Build history of the part. All positions in model axes, mm. A direction names the side the tool comes from. Coordinates: 2 decimals unless noted, no trailing zeros. Order: outer loops, then holes, each group sorted by start corner. A loop starts at its lowest first (then second) coordinate and runs counter-clockwise, first axis right, second up. Notation, with made-up numbers: (48, -22.5) - (60, -22.5) arc R24 cw to (60, 14.5) - close; hole circle Ø3 at (2, 30.5). An arc over 180 degrees is marked (long way). One line per item, written item: value.
from build123d import *

# Parameters (mm, degrees)
F1_DEPTH = 90
F2_R     = 15
F3_R     = 5


with BuildPart() as f1:
    # F0 (on Right) → F1 (new body)
    with BuildSketch(Plane.YZ):
        with BuildLine():
            Line((0, 15), (0, 0))
            Line((0, 0), (245, 0))
            Line((245, 0), (245, 50))
            Line((245, 50), (80, 50))
            Line((80, 50), (80, 75))
            ThreePointArc((80, 75), (46.6250520012, 68.4603820444), (22.3636995256, 44.6267811209))
            Line((22.3636995256, 44.6267811209), (0, 44.6267811209))
            Line((0, 44.6267811209), (0, 15))
        make_face()
    extrude(amount=F1_DEPTH)

    # F2
    f2_edges = [f1.edges().sort_by_distance(p)[0] for p in [
        (45, 0, 44.626781),
    ]]
    fillet(f2_edges, radius=F2_R)

    # F3
    f3_edges = [f1.edges().sort_by_distance(p)[0] for p in [
        (90, 46.625052, 68.460382),
        (90, 162.5, 50),
        (90, 18.68185, 44.626781),
        (45, 22.3637, 44.626781),
        (0, 18.68185, 44.626781),
        (0, 80, 62.5),
        (0, 162.5, 50),
        (45, 245, 50),
        (90, 80, 62.5),
        (45, 80, 75),
        (45, 80, 50),
        (0, 4.393398, 40.233383),
        (0, 46.625052, 68.460382),
        (0, 0, 14.813391),
        (90, 4.393398, 40.233383),
        (90, 0, 14.813391),
    ]]
    fillet(f3_edges, radius=F3_R)


solid = f1.part
1. Probe line 1 along Z through (x, y) = (77.5, 168); line 2 along X through (y, z) = (200, 48); line 3 along Y through (x, z) = (6, 53). List the from-to ranges inside material, lowest first.
Values found:
line 1: z = 0 to 50
line 2: x = 1 to 89
line 3: y = 27.94 to 80.42
2. Band-saw the part on A-A, the plane x = 30. Give the cut face in (y, z).
Values found:
outline: (0, 0) - (245, 0) - (245, 45) arc R5 ccw to (240, 50) - (85, 50) arc R5 cw to (80, 55) - (80, 70.28) arc R5 ccw to (75.07, 75.28) arc R59.17 ccw to (23.75, 47.02) arc R5 cw to (19.49, 44.63) - (15, 44.63) arc R15 ccw to (0, 29.63) - close
3. Band-saw the part on B-B, the plane y = 150.5. Give the cut face in (x, z), and give its area (3 significant figures).
Values found:
outline: (0, 0) - (90, 0) - (90, 45) arc R5 ccw to (85, 50) - (5, 50) arc R5 ccw to (0, 45) - close
area: 4,490 mm2
4. 3-axis set-ups, long thin cutter, end or side, ignore diameter. For faces 1 (the face through (1.5, 17.2, 43.2)), 2 (the face through (89, 164, 48)), 3 (the face through (44, 164, 50)), 4 (the face through (1, 164, 48)): which of +Z, -Z, +X, -X, +Y, -Y reach the whole face in a straight line?
Values found:
face 1: +Z, -X, -Y
face 2: +Z, +X, +Y
face 3: +Z, +X, -X, +Y
face 4: +Z, -X, +Y
5. Flat gauge pins, fed straight in: P1, Ø7.5, axis at x = 49, z = 61, coming from the +Y side; P2, Ø10, axis at x = 64, y = 103, coming from the -Z side; P3, Ø1.3, axis at x = 27.5, y = 18, coming from the +Z side; P4, Ø1.5, axis at x = 33.5, y = 163, coming from the +Z side. Where does each tip first touch, or does it go through?
Values found:
P1: stops at y = 80
P2: stops at z = 0
P3: stops at z = 44.63
P4: stops at z = 50
